Autodesk Inventor part; units mm, degrees
ref_plane "YZ Plane" through (0, 0, 0) normal (1, 0, 0) x (0, 1, 0)
ref_plane "XZ Plane" through (0, 0, 0) normal (0, 1, 0) x (-1, 0, 0)
ref_plane "XY Plane" through (0, 0, 0) normal (0, 0, 1) x (1, 0, 0)
sketch "Sketch1" plane through (0, 0, 0) normal (0, 1, 0) x (-1, 0, 0)
  line L0 (0, 0) -> (63.5, 0)
  line L1 (63.5, 0) -> (63.5, 50.8)
  line L2 (63.5, 50.8) -> (0, 50.8)
  line L3 (0, 50.8) -> (0, 0)
  dimension "d0" = 63.5
  dimension "d1" = 50.8
extrude "Extrusion1" add sketch "Sketch1" along normal blind 12.7
sketch "Sketch3" plane through (0, 12.7, 0) normal (0, 1, 0) x (1, 0, 0)
  circle A0 centre (-19.05, -25.4) radius 10.9093
  line L0 (-63.5, -50.8) -> (0, -50.8)
  line L1 (0, -50.8) -> (0, 0)
  dimension "d9" = 21.8186
  dimension "d22" = 19.05
  dimension "d23" = 50.8
  dimension "d24" = 25.4
extrude "Extrusion3" cut sketch "Sketch3" against normal blind 25.4
sketch "Sketch4" plane through (-63.5, 0, 50.8) normal (0, 0, 1) x (1, 0, 0)
  line L0 (0, 12.7) -> (63.5, 12.7)
  line L1 (0, 0) -> (0, 12.7)
  line L2 (0, 0) -> (5.08, 0)
  line L3 (5.08, 0) -> (5.08, 12.7)
  line L4 (5.08, 12.7) -> (0, 12.7)
  line L5 (0, 12.7) -> (0, 0)
  dimension "d12" = 5.08
extrude "Extrusion4" add sketch "Sketch4" along normal blind 12.7
sketch "Sketch5" plane through (0, 0, 0) normal (0, 0, -1) x (-1, 0, 0)
  line L0 (0, 12.7) -> (63.5, 12.7)
  line L1 (63.5, 0) -> (58.42, 0)
  line L2 (58.42, 0) -> (58.42, 12.7)
  line L3 (58.42, 12.7) -> (63.5, 12.7)
  line L4 (63.5, 12.7) -> (63.5, 0)
  dimension "d15" = 5.08
extrude "Extrusion5" add sketch "Sketch5" along normal blind 12.7
sketch "Sketch6" plane through (0, 0, 50.8) normal (1, 0, 0) x (0, 0, -1)
  line L0 (50.8, 0) -> (50.8, 12.7)
  line L1 (0, 0) -> (0, 12.7)
  circle A0 centre (6.35, 6.35) radius 3.175
  circle A1 centre (44.45, 6.35) radius 3.175
  dimension "d18" = 6.35
  dimension "d19" = 6.35
  dimension "d20" = 6.35
  dimension "d21" = 6.35
extrude "Extrusion6" cut sketch "Sketch6" against normal blind 38.1
thread "Thread1"
thread "Thread2"
sketch "Sketch7" plane through (-58.42, 0, 0) normal (1, 0, 0) x (0, 0, -1)
  circle A0 centre (6.35, 6.35) radius 3.175
  dimension "d31" = 6.35
extrude "Extrusion7" cut sketch "Sketch7" against normal blind 38.1
sketch "Sketch8" plane through (-58.42, 0, 50.8) normal (1, 0, 0) x (0, 0, -1)
  circle A0 centre (-6.35, 6.35) radius 3.175
  point P0 (50.8, 0)
  dimension "d34" = 6.35
extrude "Extrusion8" cut sketch "Sketch8" against normal blind 38.1
equation "\"d24\" = 0.5 * d23"
properties part number "Pipe bracket" material "Aluminum 6061"
For this review, take the finished solid that the model builds, in its own axes (mm). A direction names the side the tool comes from. Coordinates: 2 decimals unless noted, no trailing zeros. Loops run counter-clockwise (first coordinate to the right, second up) from the corner with the lowest first, then second, coordinate; pieces in that order, holes last. Notation, with made-up numbers: (32.5, -21) - (90.5, -21) arc R20 ccw to (90.5, -3) - close; hole circle Ø7 at (-25.5, -4.75). An arc over 180 degrees is marked (long way). Use one line per item in the form item = value. Start each with the question number.
1) Take a section at B-B (y = 6.35). State the section outline as (x, z) points (3 decimals), plus the area to 3 significant figures.
2) For faces 1 (the face through (-58.42, 3, 56)), 2 (the face through (-61, 6, -12.7)), 3 (the face through (-58.42, 3, -5)), 4 (the face through (-38.1, 6, 44)), list the 3-axis set-ups (+Z, -Z, +X, -X, +Y, -Y) from which the entire face can be reached by the end or side of a thin tool; tool diameter is ignored.
3) To check wall thickness, follow probe 1 along Z at (x, y) = (-27.5, 8.5); probe 2 along Y at (x, z) = (-26, 6); probe 3 along Z at (x, y) = (-8, 4.5). State the ranges of each line that lie inside material, in increasing order. Write a range as from..to.
4) Draft analysis for pull direction Z (two halves, no side actions). For faces 5 (the face through (-63.5, 6, 26)), 6 (the face through (-13.19, 6.44, 16.2)), 7 (the face through (-29, 6, 0)), state which applies: released by +Z, released by -Z, zero draft, split by the parting line, or undercut.
5) For pin 1 (4 mm diameter, centred on x = -23, y = 8, fed in from -Z); pin 2 (13 mm diameter, centred on x = -19.05, z = 25.4, fed in from +Y); pin 3 (1.9 mm diameter, centred on y = 5.5, z = 7.5, fed in from +X); pin 4 (6.5 mm diameter, centred on y = 7.5, z = -7, fed in from +X), all flat-tipped, find the tip position at first contact; note any pin that passes through.
6) Take a section at C-C (z = 25.4). State the section outline as (x, y) points.
7) Take a section at A-A (x = -19.05). State the section outline as (y, z) points (3 decimals), plus the area to 3 significant figures.
8) Take a section at D-D (y = 10.75). State the section outline as (x, z) points.
From the geometry:
q1.outline = (-63.5, -12.7) - (-58.42, -12.7) - (-58.42, -9.525) - (-63.5, -9.525) - close; (-63.5, -3.175) - (-58.42, -3.175) - (-58.42, 0) - (0, 0) - (0, 3.175) - (-38.1, 3.175) - (-38.1, 9.525) - (0, 9.525) - (0, 41.275) - (-38.1, 41.275) - (-38.1, 47.625) - (0, 47.625) - (0, 50.8) - (-58.42, 50.8) - (-58.42, 53.975) - (-63.5, 53.975) - close; (-63.5, 60.325) - (-58.42, 60.325) - (-58.42, 63.5) - (-63.5, 63.5) - close; hole circle Ø21.819 at (-19.05, 25.4)
q1.area = 2,430 mm2
q2.face_1 = +Z, +X, +Y, -Y
q2.face_2 = -Z, +X, -X, +Y, -Y
q2.face_3 = -Z, +X, +Y, -Y
q2.face_4 = +X
q3.probe_1 = 0..4.01, 8.69..18.5, 32.3..42.11, 46.79..50.8
q3.probe_2 = 0..3.19, 9.51..12.7
q3.probe_3 = 0..3.77, 8.93..41.87, 47.03..50.8
q4.face_5 = zero draft
q4.face_6 = undercut
q4.face_7 = released by -Z
q5.pin_1 = 0
q5.pin_2 = through
q5.pin_3 = -38.1
q5.pin_4 = -58.42
q6.outline = (-63.5, 0) - (-29.96, 0) - (-29.96, 12.7) - (-63.5, 12.7) - close; (-8.14, 0) - (0, 0) - (0, 12.7) - (-8.14, 12.7) - close
q7.outline = (0, 0) - (12.7, 0) - (12.7, 14.491) - (0, 14.491) - close; (0, 36.309) - (12.7, 36.309) - (12.7, 50.8) - (0, 50.8) - close; hole circle Ø6.35 at (6.35, 6.35); hole circle Ø6.35 at (6.35, 44.45)
q7.area = 305 mm2
q8.outline = (-63.5, -12.7) - (-58.42, -12.7) - (-58.42, 0) - (0, 0) - (0, 50.8) - (-58.42, 50.8) - (-58.42, 63.5) - (-63.5, 63.5) - close; hole circle Ø21.82 at (-19.05, 25.4)
